The listing builds one solid part. Answer for the finished solid, in the listing's coordinates (mm). Give positions to 0.01 mm unless a question says otherwise; leave off trailing zeros. Write each loop counter-clockwise with the first axis right and the second up, starting at its lowest first coordinate (ties: lowest second). Pieces come first, ordered by that corner, then holes. Notation, with made-up numbers: (7, 66) -> (24, 66) arc R24 cw to (24, 98) -> close; hole circle Ø1 at (48.5, 75.25). An arc over 180 degrees is marked (long way). Put each result on its own line as item: value. Start each with the question number.
1) Flat-ended cylindrical pins translate along their axes: pin 1 Ø6 at (x, y) = (90, -7.5) entering from +Z; pin 2 Ø12 at (y, z) = (-18, -39.5) entering from +X; pin 3 Ø2 at (y, z) = (-9.5, -22.5) entering from -X. Find the tip coordinate at first contact, or state that the pin passes through.
2) Find the intervals of material crossed by line 1 along Z through (x, y) = (84, -25); line 2 along X through (y, z) = (-12, -5); line 3 along X through (y, z) = (-4, -63), in increasing order. Write a range as from..to.
3) For a pull along Z with two mould halves and no side action, classify faces 1 (the cylindrical face through (89.26, -15.78, 37.18)), 2 (the cylindrical face through (94.966, -15.776, -24.198)), 3 (the cylindrical face through (62.944, -15.776, -74.293)), 4 (the cylindrical face through (88.61, -15.78, -22.82)) as released by +Z, released by -Z, zero draft, split by the parting line, or undercut.
4) A cutting plane is placed at A-A (y = -17). Write down the section's boundary in (x, z).
5) A cutting plane is placed at B-B (z = 10). Write down the section's boundary in (x, y).
6) A cutting plane is placed at C-C (x = 68). Write down the section's boundary in (y, z).
from build123d import *

# Parameters (mm, degrees)
F1_DEPTH = 32


with BuildPart() as f1:
    # F0 (on Front) → F1 (new body)
    with BuildSketch(Plane.XZ):
        with BuildLine():
            ThreePointArc((82.927163, 38.669571), (88.382213, -23.681943), (52.482244, -74.952412))
            Line((52.482244, -74.952412), (59.373261, -74.952412))
            ThreePointArc((59.373261, -74.952412), (62.991993, -74.274685), (66.120223, -72.333368))
            ThreePointArc((66.120223, -72.333368), (95.161877, -23.414036), (92.134269, 33.395755))
            ThreePointArc((92.134269, 33.395755), (89.206062, 37.219742), (84.613104, 38.669571))
            Line((84.613104, 38.669571), (82.927163, 38.669571))
        make_face()
    extrude(amount=F1_DEPTH)


solid = f1.part
Reply:
1. pin 1: stops at z = 38.31
1. pin 2: stops at x = 92.1
1. pin 3: stops at x = 88.43
2. line 1: z = -50.48..-36.28, 36.28..38.67
2. line 2: x = 91.36..97.87
2. line 3: x = 66.36..75.07
3. face 1: released by +Z
3. face 2: split by the parting line
3. face 3: released by -Z
3. face 4: undercut
4. outline: (52.48, -74.95) -> (59.37, -74.95) arc R10 ccw to (66.12, -72.33) arc R98 ccw to (92.13, 33.4) arc R8 ccw to (84.61, 38.67) -> (82.93, 38.67) arc R91.5 cw to start
5. outline: (90.95, -32) -> (97.49, -32) -> (97.49, 0) -> (90.95, 0) -> close
6. outline: (-32, -70.57) -> (0, -70.57) -> (0, -61.22) -> (-32, -61.22) -> close
